CAD build for the part. Positions are in the model's coordinates, mm. A direction names the side the tool comes from. Give positions to 0.01 mm unless a question says otherwise; leave off trailing zeros. Write each loop counter-clockwise with the first axis right and the second up, starting at its lowest first coordinate (ties: lowest second). Pieces come first, ordered by that corner, then holes. Notation, with made-up numbers: M -7.75,36.5 L -1.75,36.5 A31 cw -1.75,62.5 Z; hole C 44.25,65.25 d2. An arc over 180 degrees is marked long. One line per question, with ' | ' between items. Start each with the question number.
1. Cut at D-D, the plane y = 15.5. Write the cut outline in (x, z), then the cut area to 3 significant figures.
2. Wall check: L1, parallel to Z at x = 10, y = 3; L2, parallel to Y at x = 6.5, z = 4; L3, parallel to X at y = 12.25, z = 4.75. Give the ranges that are in metal, low to high.
3. Which spindle directions (+Z, -Z, +X, -X, +Y, -Y) get a long thin tool onto all of the face, cutting with end or side? Do faces 1 (the face through (0, 10.1, 0.5)), 2 (the face through (10, 15, 1)). Say none if no direction does.
4. Flat gauge pins, fed straight in: pin 1 (3 mm diameter, centred on x = 15, y = 12.5, fed in from -Z); pin 2 (1.5 mm diameter, centred on x = 3, z = 2.5, fed in from +Y); pin 3 (2 mm diameter, centred on x = 13.5, z = 6, fed in from -Y); pin 4 (1 mm diameter, centred on y = 7, z = 4.5, fed in from -X). Where does each tip first touch, or does it go through?
5. Cut at A-A, the plane x = 10. Write the cut outline in (y, z).
6. Cut at C-C, the plane z = 3. Write the cut outline in (x, y).
Autodesk Inventor part; units mm, degrees
ref_plane "YZ Plane" through (0, 0, 0) normal (1, 0, 0) x (0, 1, 0)
ref_plane "XZ Plane" through (0, 0, 0) normal (0, 1, 0) x (-1, 0, 0)
ref_plane "XY Plane" through (0, 0, 0) normal (0, 0, 1) x (1, 0, 0)
sketch "Sketch1" plane through (0, 0, 0) normal (0, 0, 1) x (1, 0, 0)
  line L0 (0, 0) -> (20, 0)
  line L1 (20, 0) -> (20, 20)
  line L2 (20, 20) -> (0, 20)
  line L3 (0, 20) -> (0, 0)
  dimension "d0" = 20
  dimension "d1" = 20
extrude "Extrusion1" add sketch "Sketch1" along normal blind 1
sketch "Sketch2" plane through (0, 0, 1) normal (0, 0, 1) x (1, 0, 0)
  line L0 (0, 20) -> (10, 20)
  line L1 (20, 20) -> (0, 20)
  line L2 (10, 20) -> (10, 10)
  circle A0 centre (10, 10) radius 4.5
  point P0 (0, 0)
  dimension "d4" = 10
  dimension "d5" = 10
  dimension "d6" = 9
extrude "Extrusion2" add sketch "Sketch2" along normal blind 7
thread "Thread1"
properties part number "crank shaft nut"
Here are the results:
1) outline: M 0,0 L 20,0 L 20,1 L 0,1 Z | area: 20.0 mm^2
2) L1: 0 to 1 | L2: 7.17 to 12.83 | L3: 6.1 to 13.9
3) face 1: +Z, -Z, -X, +Y, -Y | face 2: +Z
4) pin 1: z = 0 | pin 2: through | pin 3: y = 6.26 | pin 4: x = 6.26
5) outline: M 0,0 L 20,0 L 20,1 L 14.5,1 L 14.5,8 L 5.5,8 L 5.5,1 L 0,1 Z
6) outline: C 10,10 d9
